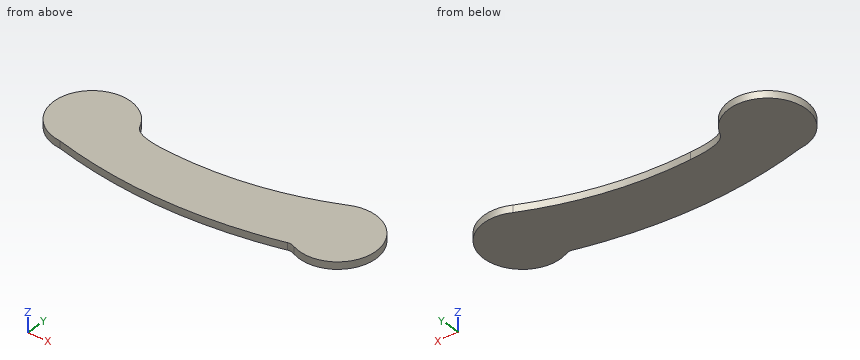
```python
from build123d import *

# Parameters (mm, degrees)
SKETCH1_R           = 5
SKETCH1_R_2         = 1.1
SKETCH1_R_3         = 4
BOSS_EXTRUDE1_DEPTH = 3


with BuildPart() as part:
    # Sketch1 → Boss-Extrude1 (new body)
    # profile 1 of 19: a face of its own
    with BuildSketch(Plane.XY):
        with BuildLine():
            ThreePointArc((68.935876888, -41.399946265), (91.352405248, -26.204284986), (67.957252813, -12.563327983))
            add(Edge.make_bspline(
                [(67.957252813, -12.563327983), (65.455609859, -13.713888582), (60.364787712, -15.882927404), (52.683559955, -18.641296662), (44.896066709, -20.933273776), (37.015370972, -22.752952432), (29.033864031, -24.103049266), (20.950849492, -24.983508442), (14.12359191, -25.325141054), (8.614596461, -25.364124484), (5.82883012, -25.303122311), (4.440642397, -25.254725163)],
                knots=[0.003418543, 0.003418543, 0.003418543, 0.003418543, 0.119867337, 0.236316132, 0.352764926, 0.46921372, 0.585662514, 0.702111309, 0.818560103, 0.8767845, 0.935008897, 0.935008897, 0.935008897, 0.935008897], degree=3))
            add(Edge.make_bspline(
                [(-11.658277887, -20.5832063), (-9.065688302, -25.060046308), (4.440642397, -25.254725163)],
                knots=[0, 0, 0, 1, 1, 1], degree=2))
            ThreePointArc((-11.658277887, -20.5832063), (-39.551034339, -17.233624375), (-27.264419704, -42.497524754))
            add(Edge.make_bspline(
                [(-27.264419704, -42.497524754), (-25.334460253, -42.955768201), (-21.452320642, -43.816124737), (-13.705385842, -45.286858174), (-4.006421964, -46.667533574), (7.638269658, -47.586831656), (19.289241844, -47.768762722), (30.941925955, -47.212824411), (42.591601286, -45.920000504), (52.298162816, -44.228522597), (60.052175742, -42.510146288), (63.940283625, -41.52535362), (65.871739475, -41.00572578)],
                knots=[0.004189422, 0.004189422, 0.004189422, 0.004189422, 0.066427583, 0.128665745, 0.253142067, 0.377618389, 0.502094711, 0.626571033, 0.751047356, 0.875523678, 0.937761839, 1, 1, 1, 1], degree=3))
            add(Edge.make_bspline(
                [(68.935876888, -41.399946265), (67.056778784, -40.529280178), (65.871739475, -41.00572578)],
                knots=[0, 0, 0, 1, 1, 1], degree=2))
        make_face()
        with Locations((75.361610976, -26.74696222)):
            Circle(SKETCH1_R, mode=Mode.SUBTRACT)
        with Locations((75.361610976, -18.74696222)):
            Circle(SKETCH1_R_2, mode=Mode.SUBTRACT)
        with Locations((81.018465226, -21.090107971)):
            Circle(SKETCH1_R_2, mode=Mode.SUBTRACT)
        with Locations((83.361610976, -26.74696222)):
            Circle(SKETCH1_R_2, mode=Mode.SUBTRACT)
        with Locations((-26.518107506, -26.514939916)):
            Circle(SKETCH1_R_3, mode=Mode.SUBTRACT)
        with Locations((81.018465226, -32.40381647)):
            Circle(SKETCH1_R_2, mode=Mode.SUBTRACT)
        with Locations((-26.516504294, -18.516504294)):
            Circle(SKETCH1_R_2, mode=Mode.SUBTRACT)
        with Locations((-20.859650045, -20.859650045)):
            Circle(SKETCH1_R_2, mode=Mode.SUBTRACT)
        with Locations((-18.516504294, -26.516504294)):
            Circle(SKETCH1_R_2, mode=Mode.SUBTRACT)
        with Locations((-20.859650045, -32.173358544)):
            Circle(SKETCH1_R_2, mode=Mode.SUBTRACT)
        with Locations((-26.516504294, -34.516504294)):
            Circle(SKETCH1_R_2, mode=Mode.SUBTRACT)
        with Locations((-32.173358544, -32.173358544)):
            Circle(SKETCH1_R_2, mode=Mode.SUBTRACT)
        with Locations((-34.516504294, -26.516504294)):
            Circle(SKETCH1_R_2, mode=Mode.SUBTRACT)
        with Locations((-32.173358544, -20.859650045)):
            Circle(SKETCH1_R_2, mode=Mode.SUBTRACT)
        with Locations((75.361610976, -34.74696222)):
            Circle(SKETCH1_R_2, mode=Mode.SUBTRACT)
        with Locations((69.704756727, -32.40381647)):
            Circle(SKETCH1_R_2, mode=Mode.SUBTRACT)
        with Locations((67.361610976, -26.74696222)):
            Circle(SKETCH1_R_2, mode=Mode.SUBTRACT)
        with Locations((69.704756727, -21.090107971)):
            Circle(SKETCH1_R_2, mode=Mode.SUBTRACT)
    # profile 2 of 19: a face of its own
    with BuildSketch(Plane.XY):
        with Locations((-20.859650045, -20.859650045)):
            Circle(SKETCH1_R_2)
    # profile 3 of 19: a face of its own
    with BuildSketch(Plane.XY):
        with Locations((-26.516504294, -18.516504294)):
            Circle(SKETCH1_R_2)
    # profile 4 of 19: a face of its own
    with BuildSketch(Plane.XY):
        with Locations((-32.173358544, -20.859650045)):
            Circle(SKETCH1_R_2)
    # profile 5 of 19: a face of its own
    with BuildSketch(Plane.XY):
        with Locations((-18.516504294, -26.516504294)):
            Circle(SKETCH1_R_2)
    # profile 6 of 19: a face of its own
    with BuildSketch(Plane.XY):
        with Locations((-20.859650045, -32.173358544)):
            Circle(SKETCH1_R_2)
    # profile 7 of 19: a face of its own
    with BuildSketch(Plane.XY):
        with Locations((-26.516504294, -34.516504294)):
            Circle(SKETCH1_R_2)
    # profile 8 of 19: a face of its own
    with BuildSketch(Plane.XY):
        with Locations((-32.173358544, -32.173358544)):
            Circle(SKETCH1_R_2)
    # profile 9 of 19: a face of its own
    with BuildSketch(Plane.XY):
        with Locations((-34.516504294, -26.516504294)):
            Circle(SKETCH1_R_2)
    # profile 10 of 19: a face of its own
    with BuildSketch(Plane.XY):
        with Locations((-26.518107506, -26.514939916)):
            Circle(SKETCH1_R_3)
    # profile 11 of 19: a face of its own
    with BuildSketch(Plane.XY):
        with Locations((83.361610976, -26.74696222)):
            Circle(SKETCH1_R_2)
    # profile 12 of 19: a face of its own
    with BuildSketch(Plane.XY):
        with Locations((81.018465226, -21.090107971)):
            Circle(SKETCH1_R_2)
    # profile 13 of 19: a face of its own
    with BuildSketch(Plane.XY):
        with Locations((75.361610976, -18.74696222)):
            Circle(SKETCH1_R_2)
    # profile 14 of 19: a face of its own
    with BuildSketch(Plane.XY):
        with Locations((69.704756727, -21.090107971)):
            Circle(SKETCH1_R_2)
    # profile 15 of 19: a face of its own
    with BuildSketch(Plane.XY):
        with Locations((67.361610976, -26.74696222)):
            Circle(SKETCH1_R_2)
    # profile 16 of 19: a face of its own
    with BuildSketch(Plane.XY):
        with Locations((69.704756727, -32.40381647)):
            Circle(SKETCH1_R_2)
    # profile 17 of 19: a face of its own
    with BuildSketch(Plane.XY):
        with Locations((75.361610976, -34.74696222)):
            Circle(SKETCH1_R_2)
    # profile 18 of 19: a face of its own
    with BuildSketch(Plane.XY):
        with Locations((81.018465226, -32.40381647)):
            Circle(SKETCH1_R_2)
    # profile 19 of 19: a face of its own
    with BuildSketch(Plane.XY):
        with Locations((75.361610976, -26.74696222)):
            Circle(SKETCH1_R)
    extrude(amount=BOSS_EXTRUDE1_DEPTH)


solid = part.part
```
Work out the finished part from the listing and answer in its coordinate system (mm). Give positions to 0.01 mm unless a question says otherwise; leave off trailing zeros. Loops run counter-clockwise (first coordinate to the right, second up) from the corner with the lowest first, then second, coordinate; pieces in that order, holes last. Notation, with made-up numbers: (-16, 35.5) -> (25, 35.5) arc R11 cw to (25, 42.5) -> close; hole circle Ø4 at (62, 57.5). An arc over 180 degrees is marked (long way). One line per question, with ' | ' between items. Start each with the question number.
1) Straight lines are drawn through the part: L1, parallel to X at y = -27, z = 0.5; L2, parallel to Y at x = -33, z = 2.35; L3, parallel to Y at x = -26, z = 2.3. For each, find the intervals that lie inside material, in ascending order.
2) This flat-tipped pin is pushed along its axis until it touches: pin 1 (1.5 mm diameter, centred on x = 13, z = 1.5, fed in from -Y). Where does it stop, or does it pass through?
3) Section B-B, the plane x = 75 is taken. Determine the outline of the cut face in (y, z).
4) Section A-A, the plane y = -35 is taken. Determine the outline of the cut face in (x, z).
Resolved:
1) L1: -42.51 to 91.36 | L2: -41.14 to -11.89 | L3: -42.79 to -10.52
2) pin 1: y = -47.65
3) outline: (-42.74, 0) -> (-10.75, 0) -> (-10.75, 3) -> (-42.74, 3) -> close
4) outline: (-40.08, 0) -> (89.07, 0) -> (89.07, 3) -> (-40.08, 3) -> close
